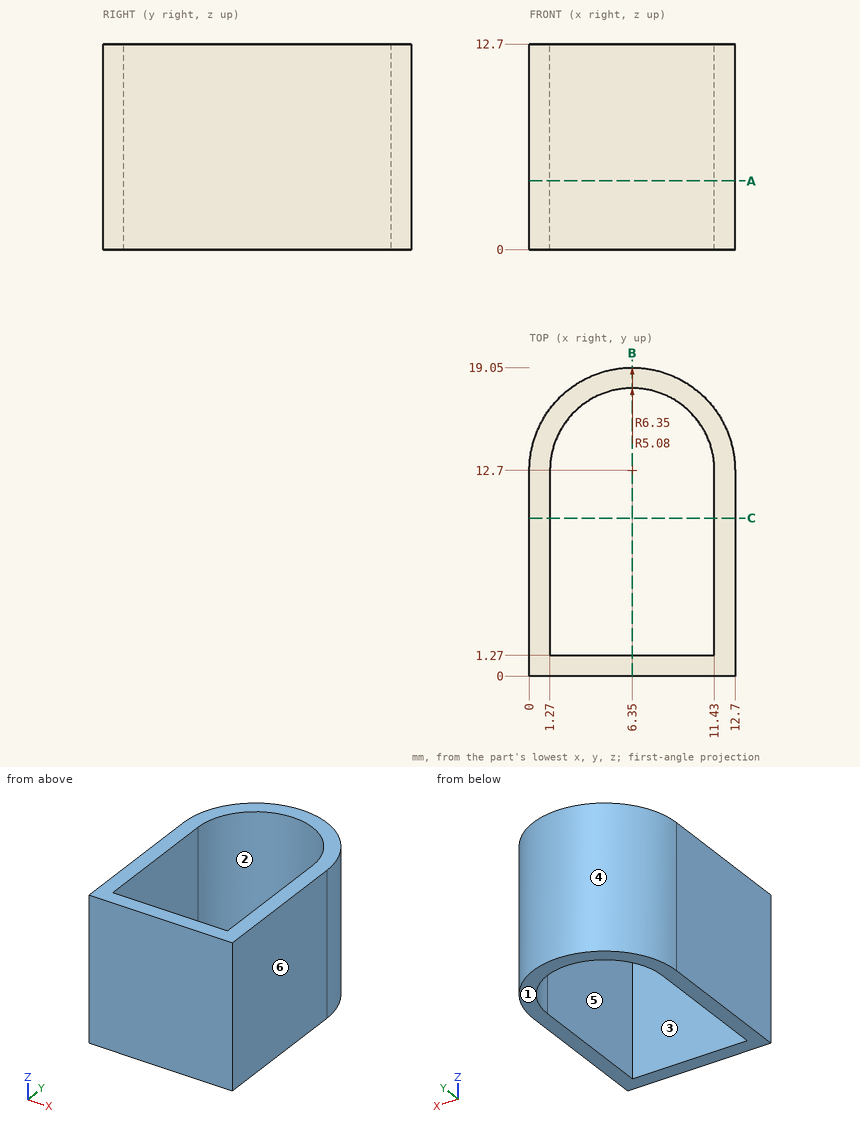
Answer from the drawing. Dimensions are ordinates in mm from the lowest x, y and z of the part. A direction names the side the tool comes from. Give positions to 0.01 mm unless a question says otherwise; leave off trailing zeros. Order: outer loops, then holes, each group sorted by start corner. A loop starts at its lowest first (then second) coordinate and runs counter-clockwise, first axis right, second up. Notation, with made-up numbers: (77.5, -1.75) - (114.5, -1.75) arc R22 cw to (114.5, 11.25) - close; hole circle Ø4 at (27.5, 23). An arc over 180 degrees is marked (long way). Use one line per item in the form item = value.
1) Find section C-C on y = 9.75. Determine the outline of the cut face in (x, z), and give its area (3 significant figures).
Verdict:
outline = (0, 0) - (1.27, 0) - (1.27, 12.7) - (0, 12.7) - close; (11.43, 0) - (12.7, 0) - (12.7, 12.7) - (11.43, 12.7) - close
area = 32.3 mm^2
2) Consider probe 1 along X at (y, z) = (9.5, 2.75); probe 2 along Y at (x, z) = (2, 5); probe 3 along Y at (x, z) = (10, 4). Determine where each line is inside the solid, lowest interval first. Write a range as [from, to].
Verdict:
probe_1 = [0, 1.27], [11.43, 12.7]
probe_2 = [0, 1.27], [15.32, 17.33]
probe_3 = [0, 1.27], [16.23, 17.9]
3) Find section B-B on x = 6.35. Determine the outline of the cut face in (y, z).
Verdict:
outline = (0, 0) - (1.27, 0) - (1.27, 12.7) - (0, 12.7) - close; (17.78, 0) - (19.05, 0) - (19.05, 12.7) - (17.78, 12.7) - close
4) Find section A-A on z = 4.25. Determine the outline of the cut face in (x, y).
Verdict:
outline = (0, 0) - (12.7, 0) - (12.7, 12.7) arc R6.35 ccw to (0, 12.7) - close; hole (1.27, 1.27) - (11.43, 1.27) - (11.43, 12.7) arc R5.08 ccw to (1.27, 12.7) - close
5) Each of these flat-tipped pins is pushed along its axis until it touches: pin 1 (2 mm diameter, centred on y = 15.5, z = 10, fed in from +X); pin 2 (4 mm diameter, centred on x = 3.5, y = 9.5, fed in from -Z); pin 3 (5 mm diameter, centred on x = 11, z = 10, fed in from +Y); pin 4 (3 mm diameter, centred on y = 15, z = 10.5, fed in from -X). Where does it stop, or does it pass through?
Verdict:
pin_1 = 12.44
pin_2 = through
pin_3 = 18.67
pin_4 = 0.05
6) The mould has two halves that part along X. Classify the marked faces 1, 2, 3 and 4: released by +X, released by -X, zero draft, split by the parting line, or undercut.
Verdict:
face_1 = zero draft
face_2 = undercut
face_3 = undercut
face_4 = split by the parting line
7) For the marked faces 5 and 6, determine the directions among +Z, -Z, +X, -X, +Y, -Y from which every point of the face is accessible in a straight line to the end or side of a thin tool.
Verdict:
face_5 = +Z, -Z
face_6 = +Z, -Z, +X, +Y, -Y
